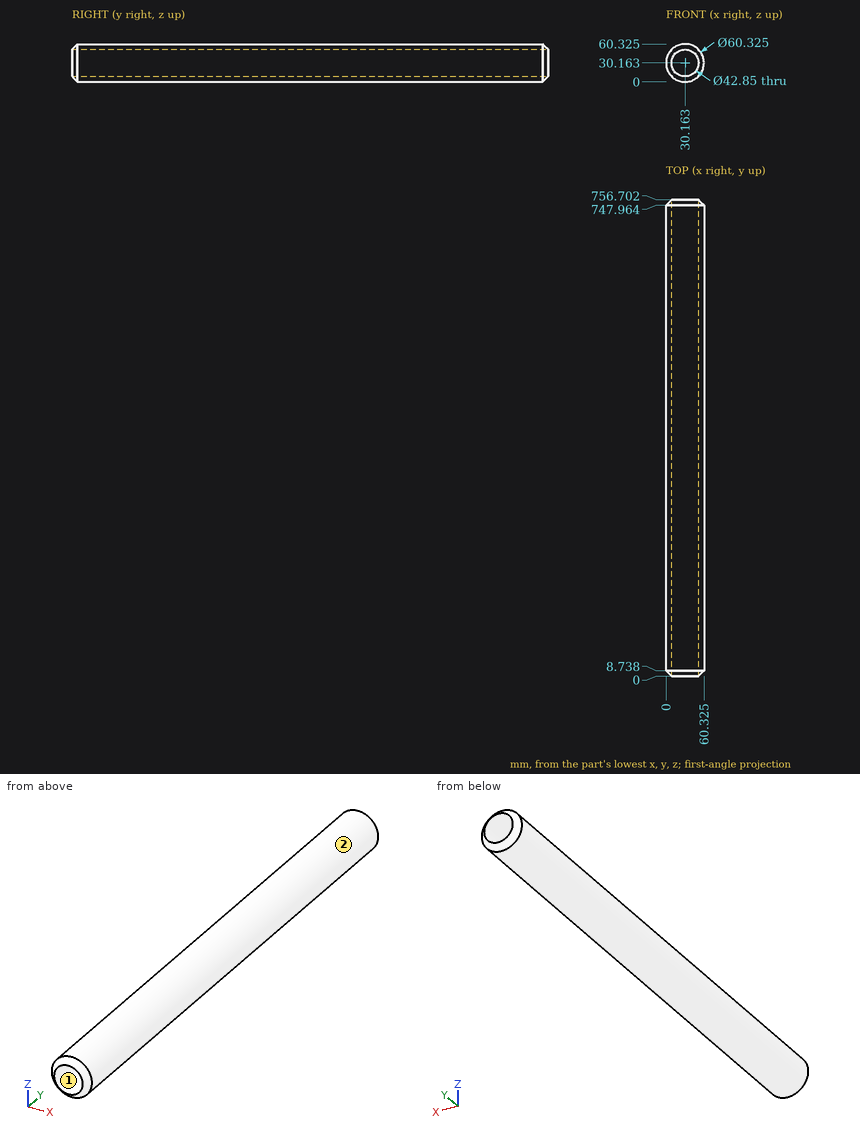
Study the drawing (mm; zero at the part's minimum x, y, z) and answer. Round coordinates to 2 decimals unless told otherwise and drop trailing zeros.
Q1. Find the intervals of material crossed by line 1 (Z direction, x = 28, y = 267.5); line 2 (X direction, y = 319, z = 12) (1 decimal); line 3 (Z direction, x = 47, y = 627) (1 decimal), in increasing order.
Q2. Given pin 1 Ø6 at (y, z) = (362.5, 44.5) entering from -X; pin 2 Ø6 at (y, z) = (603, 45.5) entering from -X; pin 3 Ø1.5 at (y, z) = (261, 53.5) entering from -X (1 decimal), each flat-ended and moving along its own axis, determine where each tip first touches the part or whether it passes through.
Q3. For a pull along X with two mould halves and no side action, classify the marked faces 1 and 2 as released by +X, released by -X, zero draft, split by the parting line, or undercut.
Completed:
1. line 1: z = 0.08 to 8.85, 51.48 to 60.25
1. line 2: x = 6.1 to 18.8, 41.5 to 54.2
1. line 3: z = 5.1 to 16.9, 43.4 to 55.2
2. pin 1: stops at x = 2.21
2. pin 2: stops at x = 2.64
2. pin 3: stops at x = 10.2
3. face 1: undercut
3. face 2: split by the parting line
